Design review of the part shown in the three views and the two pictorial views. Dimensions are in mm from the part's minimum x, y and z. A direction names the side the tool comes from. Give positions to 0.01 mm unless a question says otherwise; leave off trailing zeros. Order: outer loops, then holes, each group sorted by start corner. A loop starts at its lowest first (then second) coordinate and runs counter-clockwise, first axis right, second up. Notation, with made-up numbers: (71, -0.5) - (78, -0.5) arc R27 ccw to (78, 22.5) - close; hole circle Ø1 at (45.25, -9). An arc over 180 degrees is marked (long way). Put each result on its own line as item: value. Start each with the question number.
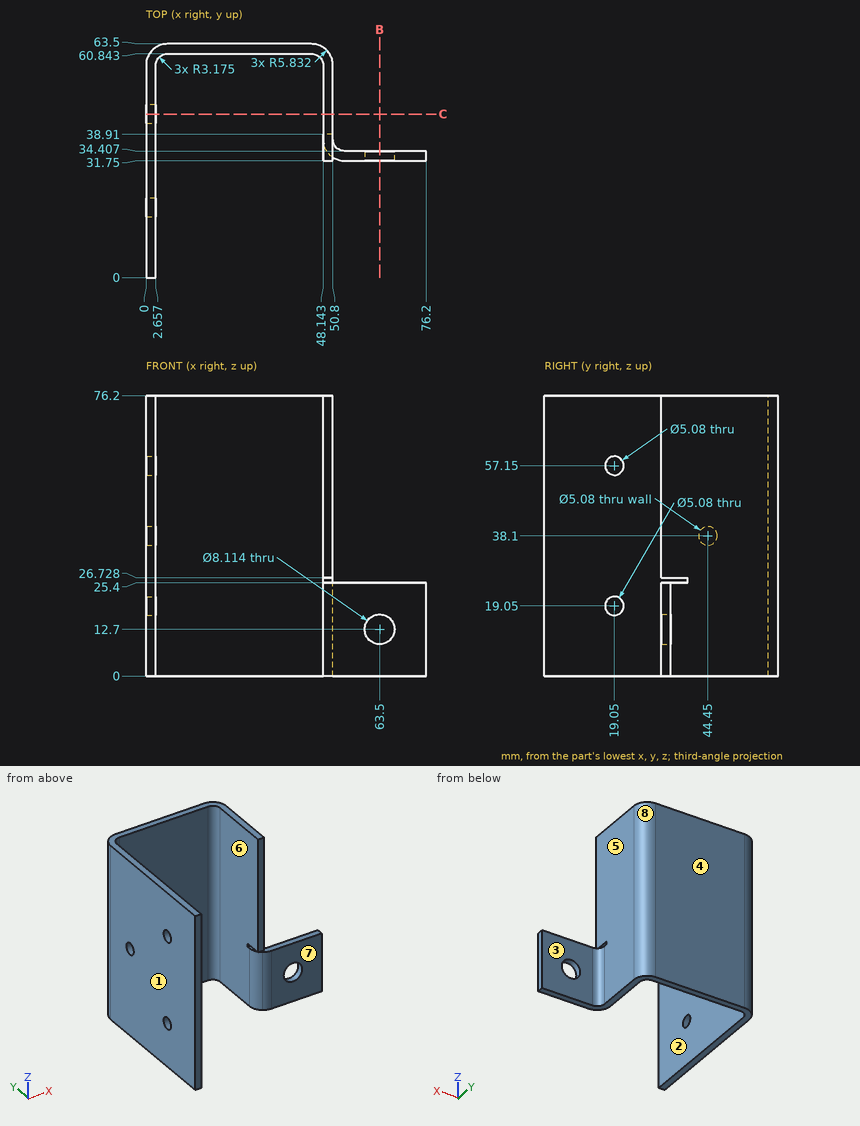
1. Tool access review of the marked faces 4, 5, 6, 7 and 8: name each direction out of +Z, -Z, +X, -X, +Y, -Y from which nothing blocks a thin tool from reaching the whole face with its end or side.
2. Clearance check with flat-ended pins moving along their axes: pin 1 (1.5 mm diameter, centred on y = 43, z = 13.5, fed in from +X); pin 2 (3 mm diameter, centred on y = 20.5, z = 29, fed in from +X); pin 3 (2 mm diameter, centred on x = 49, z = 43, fed in from -Y). State where each tip first meets the part, or that it passes through.
3. Wall thickness on line 1 (Z direction, x = 2, y = 19); line 2 (X direction, y = 45, z = 6.5); line 3 (Z direction, x = 63.5, y = 33.05): over which ranges is each line inside the solid? List them lowest first. Write a range as from..to.
4. The part is to be moulded in two halves that separate along X. For the marked faces 1, 2 and 3, say which applies: released by +X, released by -X, zero draft, split by the parting line, or undercut.
5. Add section C-C, the plane y = 44.45. Give the boundary of the cut face in (x, z).
6. Add section B-B, the plane x = 63.5. Give the boundary of the cut face in (y, z).
Found:
1. face 4: +Z, -Z, +X, -X, +Y
1. face 5: +Z, +X, +Y
1. face 6: +Z, -Z, -Y
1. face 7: +Z, -Z, +X, -Y
1. face 8: +Z, -Z, +X, +Y
2. pin 1: stops at x = 50.8
2. pin 2: stops at x = 2.66
2. pin 3: stops at y = 31.75
3. line 1: z = 0..16.51, 21.59..54.61, 59.69..76.2
3. line 2: x = 0..2.66, 48.14..50.8
3. line 3: z = 0..8.64, 16.76..25.4
4. face 1: released by -X
4. face 2: undercut
4. face 3: zero draft
5. outline: (0, 0) - (2.66, 0) - (2.66, 35.56) - (0, 35.56) - close; (0, 40.64) - (2.66, 40.64) - (2.66, 76.2) - (0, 76.2) - close; (48.14, 0) - (50.8, 0) - (50.8, 76.2) - (48.14, 76.2) - close
6. outline: (31.75, 0) - (34.41, 0) - (34.41, 8.64) - (31.75, 8.64) - close; (31.75, 16.76) - (34.41, 16.76) - (34.41, 25.4) - (31.75, 25.4) - close
